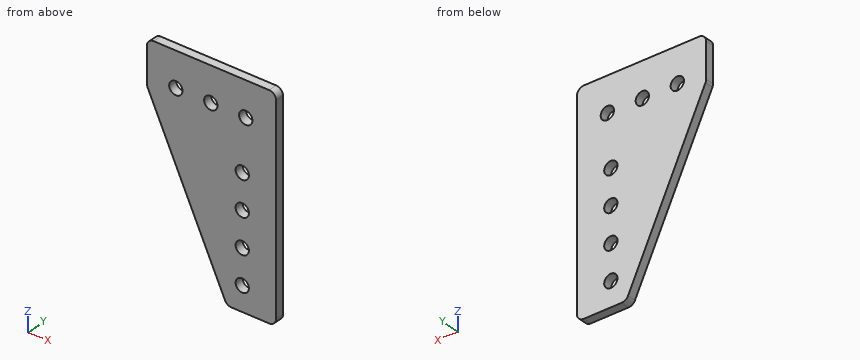
```python
from build123d import *

# Parameters (mm, degrees)
SKETCH1_W           = 50.8
SKETCH1_H           = 82.55
BOSS_EXTRUDE1_DEPTH = 3.175
SKETCH2_R           = 2.413
CUT_EXTRUDE1_DEPTH  = 97.980529618
CUT_EXTRUDE2_DEPTH  = 97.980529618
FILLET1_R           = 2.54


with BuildPart() as part:
    # Sketch1 → Boss-Extrude1 (new body)
    with BuildSketch(Plane(origin=(0, 0, 0), x_dir=(1, 0, 0), z_dir=(0, 1, 0))):
        with Locations((25.4, 41.275)):
            Rectangle(SKETCH1_W, SKETCH1_H)
    extrude(amount=BOSS_EXTRUDE1_DEPTH)

    # Sketch2 → Cut-Extrude1 (cut, through all)
    with BuildSketch(Plane(origin=(0, 3.175, 0), x_dir=(1, 0, 0), z_dir=(0, 1, 0))):
        with Locations(Location((39.752682174, 12.7, 0), (0, 0, 270))):
            Circle(SKETCH2_R)
        with Locations(Location((27.052682174, 12.7, 0), (0, 0, 270))):
            Circle(SKETCH2_R)
        with Locations(Location((14.352682174, 12.7, 0), (0, 0, 270))):
            Circle(SKETCH2_R)
        with Locations(Location((38.482682174, 31.75, 0), (0, 0, 270))):
            Circle(SKETCH2_R)
        with Locations(Location((38.482682174, 44.45, 0), (0, 0, 270))):
            Circle(SKETCH2_R)
        with Locations(Location((38.482682174, 57.15, 0), (0, 0, 270))):
            Circle(SKETCH2_R)
        with Locations(Location((38.482682174, 69.85, 0), (0, 0, 270))):
            Circle(SKETCH2_R)
    extrude(amount=-CUT_EXTRUDE1_DEPTH, mode=Mode.SUBTRACT)

    # Sketch3 → Cut-Extrude2 (cut, through all)
    with BuildSketch(Plane(origin=(0, 3.175, 0), x_dir=(1, 0, 0), z_dir=(0, 1, 0))):
        Polygon((3.859765226, 0), (3.859765226, 15.946793053), (32.906889952, 78.808591348), (50.8, 78.808591348), (50.8, 82.55), (0, 82.55), (0, 0), align=None)
    extrude(amount=-CUT_EXTRUDE2_DEPTH, mode=Mode.SUBTRACT)

    # Fillet1
    fillet1_edges = [part.edges().sort_by_distance(p)[0] for p in [
        (3.859765226, 1.5875, 0),
        (50.8, 1.5875, -78.808591348),
        (32.906889952, 1.5875, -78.808591348),
        (3.859765226, 1.5875, -15.946793053),
        (50.8, 1.5875, 0),
    ]]
    fillet(fillet1_edges, radius=FILLET1_R)


solid = part.part
```
Here's how the part is built. I have some questions about the finished solid (model axes, mm). Give positions to 0.01 mm unless a question says otherwise; leave off trailing zeros. Loops run counter-clockwise (first coordinate to the right, second up) from the corner with the lowest first, then second, coordinate; pieces in that order, holes last. Notation, with made-up numbers: M -3,75.25 L 6,75.25 A26 cw 6,107.25 Z; hole C 20.5,-32.5 d10. An arc over 180 degrees is marked long. Return JSON: item names as keys, results as strings.
Item 1: Imagine slicing it at D-D on z = -31.75. List the corners of the cut face in (x, y) for me (3 decimals).
A:
{"outline": "M 11.162,0 L 36.07,0 L 36.07,3.175 L 11.162,3.175 Z; M 40.896,0 L 50.8,0 L 50.8,3.175 L 40.896,3.175 Z"}
Item 2: Imagine slicing it at B-B on z = -57.15. List the corners of the cut face in (x, y) for me (3 decimals), then the cut area to 3 significant figures.
A:
{"outline": "M 22.899,0 L 36.07,0 L 36.07,3.175 L 22.899,3.175 Z; M 40.896,0 L 50.8,0 L 50.8,3.175 L 40.896,3.175 Z", "area": "73.3 mm^2"}
Item 3: Imagine slicing it at C-C on y = 1.55. List the corners of the cut face in (x, z) for me.
A:
{"outline": "M 3.86,-15.39 A2.54 ccw 4.09,-16.45 L 32.23,-77.33 A2.54 ccw 34.53,-78.81 L 48.26,-78.81 A2.54 ccw 50.8,-76.27 L 50.8,-2.54 A2.54 ccw 48.26,0 L 6.4,0 A2.54 ccw 3.86,-2.54 Z; hole C 14.35,-12.7 d4.83; hole C 27.05,-12.7 d4.83; hole C 38.48,-69.85 d4.83; hole C 38.48,-57.15 d4.83; hole C 38.48,-44.45 d4.83; hole C 38.48,-31.75 d4.83; hole C 39.75,-12.7 d4.83"}
Item 4: I'm going to push a flat-ended pin straight in: pin 1 Ø6.5 at (x, z) = (27.05, -12.7) entering from -Y. Where does the tip first touch, or does it pass through?
A:
{"pin 1": "stops at y = 0"}
Item 5: Please list where these lines run through material, in increasing order: line 1 (X direction, y = 1.9, z = -12.7); line 2 (X direction, y = 0.9, z = -11); line 3 (Z direction, x = 39, y = 3.05).
A:
{"line 1": "x = 3.86 to 11.94, 16.77 to 24.64, 29.47 to 37.34, 42.17 to 50.8", "line 2": "x = 3.86 to 12.64, 16.07 to 25.34, 28.77 to 38.04, 41.47 to 50.8", "line 3": "z = -78.81 to -72.21, -67.49 to -59.51, -54.79 to -46.81, -42.09 to -34.11, -29.39 to -14.99, -10.41 to 0"}
Item 6: Imagine slicing it at A-A on z = -12.7. List the corners of the cut face in (x, y) for me (3 decimals).
A:
{"outline": "M 3.86,0 L 11.94,0 L 11.94,3.175 L 3.86,3.175 Z; M 16.766,0 L 24.64,0 L 24.64,3.175 L 16.766,3.175 Z; M 29.466,0 L 37.34,0 L 37.34,3.175 L 29.466,3.175 Z; M 42.166,0 L 50.8,0 L 50.8,3.175 L 42.166,3.175 Z"}
